Here's how the part is built. I have some questions about the finished solid (model axes, mm). Coordinates: 2 decimals unless noted, no trailing zeros. Write each loop counter-clockwise with the first axis right and the second up, starting at its lowest first coordinate (ties: lowest second). Pieces come first, ordered by that corner, then holes. Notation, with made-up numbers: (-5.75, -0.75) -> (6.25, -0.75) arc R28 cw to (6.25, 28.25) -> close; hole circle Ø6 at (-20, 77.25). An arc over 180 degrees is marked (long way). Put each result on its own line as item: value.
```python
from build123d import *

# Parameters (mm, degrees)
F0_W     = 49.041539
F0_H     = 47.77154
F0_R     = 16.952149
F1_DEPTH = 63.72292
F2_R     = 5.08
F3_R     = 1.27


with BuildPart() as f1:
    # F0 (on Front) → F1 (new body)
    with BuildSketch(Plane.XZ):
        with Locations((24.52077, 23.88577)):
            Rectangle(F0_W, F0_H)
        with Locations((24.52077, 23.88577)):
            Circle(F0_R, mode=Mode.SUBTRACT)
    extrude(amount=F1_DEPTH)

    # F2
    f2_edges = [f1.edges().sort_by_distance(p)[0] for p in [
        (49.041539, -31.86146, 47.77154),
        (0, -31.86146, 47.77154),
        (49.041539, -31.86146, 0),
        (0, -31.86146, 0),
    ]]
    fillet(f2_edges, radius=F2_R)

    # F3
    f3_edges = [f1.edges().sort_by_distance(p)[0] for p in [
        (49.041539, -63.72292, 23.88577),
    ]]
    fillet(f3_edges, radius=F3_R)


solid = f1.part
```
Item 1: Please list where these lines run through material, in increasing order: line 1 along X through (y, z) = (-44, 23.5); line 2 along X through (y, z) = (-27.5, 5); line 3 along Z through (x, y) = (21.5, -33). Write a range as from..to.
Output:
line 1: x = 0..7.57, 41.47..49.04
line 2: x = 0..49.04
line 3: z = 0..7.2, 40.57..47.77
Item 2: For P1, Ø2, axis at x = 24.5, z = 39.5, coming from the +Y side, with a flat end and sliding along its axis, tell me the tip position at first contact or that it passes through.
Output:
P1: passes through
Item 3: If we mould it in two halves opening along Z, with no side actions, what happens to faces 1 (the flat face through (24, -31, 47.772)), 2 (the flat face through (24, -31, 0)), 3 (the cylindrical face through (22.314, -31.415, 40.694)), 4 (the flat face through (18.7, 0, 40.1))? For each: released by +Z, released by -Z, zero draft, split by the parting line, or undercut.
Output:
face 1: released by +Z
face 2: released by -Z
face 3: undercut
face 4: zero draft
Item 4: Imagine slicing it at C-C on y = -45.5. Write out the boundary of the cut face in (x, z), then the cut area to 3 significant figures.
Output:
outline: (0, 5.08) arc R5.08 ccw to (5.08, 0) -> (43.96, 0) arc R5.08 ccw to (49.04, 5.08) -> (49.04, 42.69) arc R5.08 ccw to (43.96, 47.77) -> (5.08, 47.77) arc R5.08 ccw to (0, 42.69) -> close; hole circle Ø33.9 at (24.52, 23.89)
area: 1,420 mm²
Item 5: Imagine slicing it at A-A on z = 16. Write out the boundary of the cut face in (x, y), then the cut area to 3 significant figures.
Output:
outline: (0, -62.45) arc R1.27 ccw to (1.27, -63.72) -> (9.51, -63.72) -> (9.51, 0) -> (0, 0) -> close; (39.53, -63.72) -> (47.77, -63.72) arc R1.27 ccw to (49.04, -62.45) -> (49.04, 0) -> (39.53, 0) -> close
area: 1,210 mm²
Item 6: Imagine slicing it at B-B on x = 9.5. Write out the boundary of the cut face in (y, z).
Output:
outline: (-63.72, 1.27) arc R1.27 ccw to (-62.45, 0) -> (0, 0) -> (0, 16.03) -> (-63.72, 16.03) -> close; (-63.72, 31.74) -> (0, 31.74) -> (0, 47.77) -> (-62.45, 47.77) arc R1.27 ccw to (-63.72, 46.5) -> close
